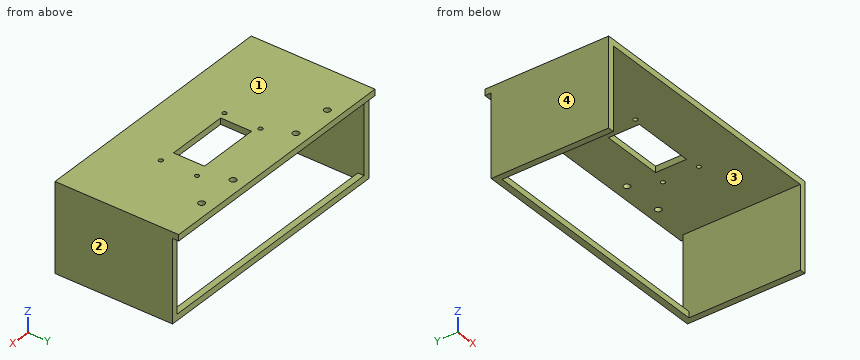
from build123d import *

# Parameters (mm, degrees)
SKETCH_1_W      = 125
SKETCH_1_H      = 60
SKETCH_1_R      = 1.55
SKETCH_1_R_2    = 1.05
SKETCH_1_W_2    = 30
SKETCH_1_H_2    = 15
EXTRUDE_1_DEPTH = 3
SKETCH_4_W      = 3
SKETCH_4_H      = 57
EXTRUDE_3_DEPTH = 43
SKETCH_6_W      = 125
SKETCH_6_H      = 3
EXTRUDE_5_DEPTH = 3


with BuildPart() as part:
    # 草图1 → 凸台-拉伸1 (new body)
    with BuildSketch(Plane.XY):
        Rectangle(SKETCH_1_W, SKETCH_1_H)
        with Locations((-40, 24)):
            Circle(SKETCH_1_R, mode=Mode.SUBTRACT)
        with Locations((-20, 24)):
            Circle(SKETCH_1_R, mode=Mode.SUBTRACT)
        with Locations((20, 24)):
            Circle(SKETCH_1_R, mode=Mode.SUBTRACT)
        with Locations((40, 24)):
            Circle(SKETCH_1_R, mode=Mode.SUBTRACT)
        with Locations((-14.25, 11.25)):
            Circle(SKETCH_1_R_2, mode=Mode.SUBTRACT)
        with Locations((-14.25, -6.25)):
            Circle(SKETCH_1_R_2, mode=Mode.SUBTRACT)
        with Locations((26.25, 11.25)):
            Circle(SKETCH_1_R_2, mode=Mode.SUBTRACT)
        with Locations((26.25, -6.25)):
            Circle(SKETCH_1_R_2, mode=Mode.SUBTRACT)
        with Locations((4.25, 2.05)):
            Rectangle(SKETCH_1_W_2, SKETCH_1_H_2, mode=Mode.SUBTRACT)
    extrude(amount=EXTRUDE_1_DEPTH)

    # 草图4 → 凸台-拉伸3 (add)
    with BuildSketch(Plane.XY.offset(3)):
        with Locations((-61, -1.5)):
            Rectangle(SKETCH_4_W, SKETCH_4_H)
        with Locations((61, -1.5)):
            Rectangle(SKETCH_4_W, SKETCH_4_H)
    extrude(amount=-EXTRUDE_3_DEPTH)

    # 草图6 → 凸台-拉伸5 (add)
    with BuildSketch(Plane(origin=(0, 27, 0), x_dir=(1, 0, 0), z_dir=(0, 1, 0))):
        with Locations((0, 38.5)):
            Rectangle(SKETCH_6_W, SKETCH_6_H)
    extrude(amount=-EXTRUDE_5_DEPTH)


solid = part.part
Could you check a few things on this model? Use its own coordinates, in mm. Face numbers are marked on the shaded views. Give positions to 0.01 mm unless a question says otherwise; leave off trailing zeros. Order: outer loops, then holes, each group sorted by start corner. A loop starts at its lowest first (then second) coordinate and runs counter-clockwise, first axis right, second up.
Item 1: If we mould it in two halves opening along X, with no side actions, what happens to the marked faces 1, 2, 3 and 4? For each: pulls with the +X half, pulls with the -X half, needs draft (parallel to the pull), parting line crosses it, or undercut.
Item 2: I need wall thicknesses on line 1 (Y direction, x = -40, z = 0.8); line 2 (X direction, y = -1.5, z = -30.5); line 3 (Y direction, x = -14, z = 1). Which ranges of each line are inside material? Lowest first, please.
Item 3: If we section it at B-B, the plane z = -4.5: Write out the boundary of the cut face in (x, y).
Item 4: If we section it at D-D, the plane y = -12.5: Write out the boundary of the cut face in (x, z), plus the area to 3 significant figures.
Item 5: If we section it at A-A, the plane x = 31.5: Write out the boundary of the cut face in (y, z).
Item 6: I'm going to push flat-ended pins straight in: pin 1 (4 mm diameter, centred on x = 10, y = 21.5, fed in from -Z); pin 2 (2.5 mm diameter, centred on x = 40, y = 24, fed in from +Z). Where does each tip first touch, or does it pass through?
Item 7: If we section it at C-C, the plane x = 15.5: Write out the boundary of the cut face in (y, z).
Values:
1. face 1: needs draft
1. face 2: pulls with the +X half
1. face 3: undercut
1. face 4: pulls with the -X half
2. line 1: y = -30 to 22.45, 25.55 to 30
2. line 2: x = -62.5 to -59.5, 59.5 to 62.5
2. line 3: y = -30 to -7.27, -5.23 to 10.23, 12.27 to 30
3. outline: (-62.5, -30) - (-59.5, -30) - (-59.5, 27) - (-62.5, 27) - close; (59.5, -30) - (62.5, -30) - (62.5, 27) - (59.5, 27) - close
4. outline: (-62.5, -40) - (-59.5, -40) - (-59.5, 0) - (59.5, 0) - (59.5, -40) - (62.5, -40) - (62.5, 3) - (-62.5, 3) - close
4. area: 615 mm2
5. outline: (-30, 0) - (30, 0) - (30, 3) - (-30, 3) - close; (24, -40) - (27, -40) - (27, -37) - (24, -37) - close
6. pin 1: stops at z = 0
6. pin 2: stops at z = -37
7. outline: (-30, 0) - (-5.45, 0) - (-5.45, 3) - (-30, 3) - close; (9.55, 0) - (30, 0) - (30, 3) - (9.55, 3) - close; (24, -40) - (27, -40) - (27, -37) - (24, -37) - close
